Source: CAD feature listing. Evaluate the final solid. Frame: model axes, mm. A direction names the side the tool comes from. Coordinates: 2 decimals unless noted, no trailing zeros. Order: outer loops, then holes, each group sorted by start corner. A loop starts at its lowest first (then second) coordinate and runs counter-clockwise, first axis right, second up.
Item 1: Section B-B on x = 22.5. Return the cut outline in (y, z), then the cut area to 3 significant figures.
Item 2: Contact query for flat-ended pins moving along their axis: P1, Ø13.5, axis at x = 21, z = -13, coming from the -Y side; P2, Ø2, axis at x = 13, z = 8, coming from the +Y side; P3, Ø5, axis at x = 40, z = 8.5, coming from the +Y side. Output: stop coordinate, or through.
Item 3: Section C-C on y = -7.5. Return the cut outline in (x, z), then the cut area to 3 significant figures.
Item 4: Ray query, line 1 (X direction, y = -2.6, z = 8.5); line 2 (X direction, y = -5.45, z = 8.5); line 3 (Z direction, x = 5, y = -6). Return the intervals inside material, ascending.
Item 5: Section A-A on z = -13. Return the cut outline in (x, y).
Item 6: Section D-D on z = 8.5. Return the cut outline in (x, y), then the cut area to 3 significant figures.
Item 7: Reachability of faces 1 (the flat face through (22, -1.5, 8)), 2 (the flat face through (4, -4.5, 7)), 3 (the flat face through (23, -5.5, -17)) from +Z, -Z, +X, -X, +Y, -Y: full face, straight path, thin tool, end or side. Return the list, or none.
Item 8: Mould query, pull axis X, two halves, no side actions, for faces 4 (the flat face through (23, -8.5, -3)), 5 (the flat face through (45, -3, -8)), 6 (the flat face through (0, -3, -8)), 7 (the cylindrical face through (4.65, -6.47, 6.94)). Classes: released by +X, released by -X, zero draft, split by the parting line, or undercut.
from build123d import *

# Parameters (mm, degrees)
ESBO_O1_W                  = 90
ESBO_O1_H                  = 3
RESSALTO_EXTRUS_O1_DEPTH   = 4
ESBO_O2_W                  = 45
ESBO_O2_H                  = 13
ESBO_O2_R                  = 1.6
RESSALTO_EXTRUS_O3_DEPTH   = 7
CORTE_EXTRUS_O1_DEPTH      = 10
CORTE_EXTRUS_O1_DEPTH_BACK = 3
ESBO_O3_R                  = 3.1
FILETE3_R                  = 2
ESBO_O4_W                  = 45
ESBO_O4_H                  = 3
CORTE_EXTRUS_O2_DEPTH      = 47.671726032
ESBO_O5_W                  = 30
ESBO_O5_H                  = 10
RESSALTO_EXTRUS_O4_DEPTH   = 45
ESBO_O6_R                  = 3.25
CORTE_EXTRUS_O3_DEPTH      = 56.000000082
ESBO_O7_R                  = 8.5
CORTE_EXTRUS_O5_DEPTH      = 3


with BuildPart() as part:
    # Esboço1 → Ressalto-extrusão1 (new body)
    with BuildSketch(Plane.XY):
        Rectangle(ESBO_O1_W, ESBO_O1_H)
    extrude(amount=RESSALTO_EXTRUS_O1_DEPTH)

    # Esboço2 → Ressalto-extrusão3 (add)
    with BuildSketch(Plane.XZ.offset(1.5)):
        with Locations((22.5, 6.5)):
            Rectangle(ESBO_O2_W, ESBO_O2_H)
        with Locations((40, 8.5)):
            Circle(ESBO_O2_R, mode=Mode.SUBTRACT)
        with Locations((5, 8.5)):
            Circle(ESBO_O2_R, mode=Mode.SUBTRACT)
    extrude(amount=RESSALTO_EXTRUS_O3_DEPTH)

    # Esboço3 → Corte-extrusão1 (cut, two sides: drawn at the far end of the back side and taken through both)
    with BuildSketch(Plane(origin=(0, -1.5, 0), x_dir=(1, 0, 0), z_dir=(0, 1, 0)).offset(-CORTE_EXTRUS_O1_DEPTH_BACK)):
        with Locations(Location((5, -8.5, 0), (0, 0, 180))):
            Circle(ESBO_O3_R)
        with Locations(Location((40, -8.5, 0), (0, 0, 180))):
            Circle(ESBO_O3_R)
    extrude(amount=CORTE_EXTRUS_O1_DEPTH + CORTE_EXTRUS_O1_DEPTH_BACK, mode=Mode.SUBTRACT)

    # Filete3
    # the kernel refuses this fillet: 2 mm, written as the material it takes off along each edge
    with BuildSketch(Plane(origin=(50, -1.5, 13), x_dir=(0, 0, -1), z_dir=(-1, 0, 0))) as filete3_piece_1:
        with BuildLine():
            CenterArc((FILETE3_R, FILETE3_R), FILETE3_R, 180, 90)
            Line((0, FILETE3_R), (0, 0))
            Line((0, 0), (FILETE3_R, 0))
        make_face()
    extrude(amount=55, mode=Mode.SUBTRACT)

    # Esboço4 → Corte-extrusão2 (cut, through all)
    with BuildSketch(Plane.XY.offset(4)):
        with Locations((-22.5, 0)):
            Rectangle(ESBO_O4_W, ESBO_O4_H)
    extrude(amount=-CORTE_EXTRUS_O2_DEPTH, mode=Mode.SUBTRACT)

    # Esboço5 → Ressalto-extrusão4 (add)
    with BuildSketch(Plane(origin=(45, 0, 0), x_dir=(0, 0, -1), z_dir=(1, 0, 0))):
        with Locations((15, -3.5)):
            Rectangle(ESBO_O5_W, ESBO_O5_H)
    extrude(amount=-RESSALTO_EXTRUS_O4_DEPTH)

    # Esboço6 → Corte-extrusão3 (cut, through all)
    with BuildSketch(Plane.XZ.offset(8.5)):
        with Locations((22.5, -13)):
            Circle(ESBO_O6_R)
    extrude(amount=-CORTE_EXTRUS_O3_DEPTH, mode=Mode.SUBTRACT)

    # Esboço7 → Corte-extrusão5 (cut)
    with BuildSketch(Plane(origin=(0, -8.5, 0), x_dir=(1, 0, 0), z_dir=(0, 1, 0))):
        with Locations(Location((22.5, 13, 0), (0, 0, 180))):
            Circle(ESBO_O7_R)
    extrude(amount=CORTE_EXTRUS_O5_DEPTH, mode=Mode.SUBTRACT)


solid = part.part
Answer list:
1. outline: (-8.5, -30) - (1.5, -30) - (1.5, -16.25) - (-5.5, -16.25) - (-5.5, -21.5) - (-8.5, -21.5) - close; (-8.5, -4.5) - (-5.5, -4.5) - (-5.5, -9.75) - (1.5, -9.75) - (1.5, 4) - (-1.5, 4) - (-1.5, 11) arc R2 ccw to (-3.5, 13) - (-8.5, 13) - close
1. area: 306 mm2
2. P1: stops at y = -5.5
2. P2: stops at y = -1.5
2. P3: stops at y = -4.5
3. outline: (0, -30) - (45, -30) - (45, 13) - (0, 13) - close; hole circle Ø3.2 at (5, 8.5); hole circle Ø17 at (22.5, -13); hole circle Ø3.2 at (40, 8.5)
3. area: 1,690 mm2
4. line 1: x = 0 to 1.9, 8.1 to 36.9, 43.1 to 45
4. line 2: x = 0 to 3.4, 6.6 to 38.4, 41.6 to 45
4. line 3: z = -30 to 6.9, 10.1 to 13
5. outline: (0, -8.5) - (14, -8.5) - (14, -5.5) - (19.25, -5.5) - (19.25, 1.5) - (0, 1.5) - close; (25.75, -5.5) - (31, -5.5) - (31, -8.5) - (45, -8.5) - (45, 1.5) - (25.75, 1.5) - close
6. outline: (0, -8.5) - (3.4, -8.5) - (3.4, -4.5) - (1.9, -4.5) - (1.9, -1.5) - (0, -1.5) - close; (6.6, -8.5) - (38.4, -8.5) - (38.4, -4.5) - (36.9, -4.5) - (36.9, -1.5) - (8.1, -1.5) - (8.1, -4.5) - (6.6, -4.5) - close; (41.6, -8.5) - (45, -8.5) - (45, -1.5) - (43.1, -1.5) - (43.1, -4.5) - (41.6, -4.5) - close
6. area: 252 mm2
7. face 1: +Z, +X, -X, +Y
7. face 2: +Y
7. face 3: -Y
8. face 4: zero draft
8. face 5: released by +X
8. face 6: released by -X
8. face 7: undercut
